Autodesk Inventor part; units mm, degrees
ref_plane "YZ Plane" through (0, 0, 0) normal (1, 0, 0) x (0, 1, 0)
ref_plane "XZ Plane" through (0, 0, 0) normal (0, 1, 0) x (-1, 0, 0)
ref_plane "XY Plane" through (0, 0, 0) normal (0, 0, 1) x (1, 0, 0)
sketch "Sketch1" plane through (0, 0, 0) normal (0, 0, 1) x (1, 0, 0)
  circle A0 centre (-18.3721, 25.1477) radius 2.1844
  circle A1 centre (57.8279, 25.1477) radius 2.1844
  circle A2 centre (32.4279, -12.9523) radius 2.1844
  circle A3 centre (-56.4721, -12.9523) radius 2.1844
  arc A4 (-60.9623, -8.4622) -> (-56.4721, -19.3023) centre (-56.4721, -12.9523) ccw
  arc A5 (-18.3721, 31.4977) -> (-22.8623, 29.6378) centre (-18.3721, 25.1477) ccw
  line L0 (68.9404, 23.5133) -> (68.9404, 25.1477)
  line L1 (62.5904, 31.4977) -> (57.8279, 31.4977)
  arc A6 (68.9404, 25.1477) -> (62.5904, 31.4977) centre (62.5904, 25.1477) ccw
  line L2 (-3.5614, -19.3023) -> (-56.4721, -19.3023)
  line L3 (-60.9623, -8.4622) -> (-22.8623, 29.6378)
  line L4 (-18.3721, 31.4977) -> (57.8279, 31.4977)
  arc A7 (35.7428, -27.2531) -> (68.9404, 23.5133) centre (13.525, 23.5133) ccw
  line L5 (29.3044, -27.6849) -> (3.4241, -20.2818)
  arc A8 (29.3044, -27.6849) -> (35.7428, -27.2531) centre (31.9239, -18.5272) ccw
  arc A9 (3.4241, -20.2818) -> (-3.5614, -19.3023) centre (-3.5614, -44.7023) ccw
  point P0 (0, 0)
  point P1 (32.4279, -28.5784)
  dimension "d0" = 4.3688
  dimension "d1" = 12.7
  dimension "d2" = 12.7
  dimension "d4" = 6.35
  dimension "d21" = 9.525
  dimension "d22" = 25.4
extrude "Extrusion1" add sketch "Sketch1" along normal blind 1.5875
sketch "Sketch2" plane through (0, 0, 1.5875) normal (0, 0, 1) x (1, 0, 0)
  circle A0 centre (57.15, 0) radius 2.0828
  point P0 (0, 0)
  dimension "d7" = 4.1656
extrude "Extrusion2" cut sketch "Sketch2" against normal blind 1.5875
sketch "Sketch3" plane through (57.8279, 25.1477, 1.5875) normal (0, 0, 1) x (1, 0, 0)
  circle A0 centre (-50.8, 25.4) radius 2.0828
  arc A1 (-45.3375, 28.6378) -> (-55.2901, 29.8901) centre (-50.8, 25.4) ccw
  line L0 (-80.6901, 4.4901) -> (-55.2901, 29.8901)
  arc A2 (-76.2, 6.35) -> (-80.6901, 4.4901) centre (-76.2, 0) ccw
  arc A3 (-45.3375, 28.6378) -> (-6.2178, 6.35) centre (-6.2178, 51.8254) ccw
  line L1 (4.7625, 6.35) -> (-76.2, 6.35)
  dimension "d17" = 4.1656
extrude "Extrusion4" add sketch "Sketch3" against normal blind 1.5875
properties part number "sled" material "Acetal Resin, White"
Input: part model. Units: mm. Frame: model coordinates. Coordinates: 2 decimals unless noted, no trailing zeros. Loops run counter-clockwise (first coordinate to the right, second up) from the corner with the lowest first, then second, coordinate; pieces in that order, holes last.
Q1. Section C-C, the plane y = 0. Return the cut outline in (x, z).
Results are:
outline: (-52.5, 0) - (55.07, 0) - (55.07, 1.59) - (-52.5, 1.59) - close; (59.23, 0) - (63.7, 0) - (63.7, 1.59) - (59.23, 1.59) - close
Q2. Line query: line 1 along X through (y, z) = (26.5, 1.3); line 2 along Y through (x, z) = (-17.5, 1.1); line 3 along X through (y, z) = (50.5, 0.6). Output: solid intervals per line, ascending.
Results are:
line 1: x = -26 to -20.09, -16.66 to 56.11, 59.54 to 68.79
line 2: y = -19.3 to 23.14, 27.15 to 35
line 3: x = -2 to 4.95, 9.11 to 14.63
Q3. Section A-A, the plane x = 57.15. Return the cut outline in (y, z).
Results are:
outline: (-10.66, 0) - (-2.08, 0) - (-2.08, 1.59) - (-10.66, 1.59) - close; (2.08, 0) - (23.07, 0) - (23.07, 1.59) - (2.08, 1.59) - close; (27.22, 0) - (31.5, 0) - (31.5, 1.59) - (27.22, 1.59) - close
Q4. Mould query, pull axis X, two halves, no side actions, for faces 1 (the cylindrical face through (28.813, 37.625, 0.805)), 2 (the cylindrical face through (-62.298, -15.479, 0.783)), 3 (the cylindrical face through (55.07, 0.09, 0.8)). Classes: +X half, -X half, draft (parallel to the pull), parting line (faces both ways), or undercut.
Results are:
face 1: +X half
face 2: -X half
face 3: undercut
Q5. Section B-B, the plane z = 1.3. Return the cut outline in (x, y).
Results are:
outline: (-60.96, -8.46) arc R6.35 ccw to (-56.47, -19.3) - (-3.56, -19.3) arc R25.4 cw to (3.42, -20.28) - (29.3, -27.68) arc R9.53 ccw to (35.74, -27.25) arc R55.42 ccw to (68.94, 23.51) - (68.94, 25.15) arc R6.35 ccw to (62.59, 31.5) - (51.61, 31.5) arc R45.48 cw to (12.49, 53.79) arc R6.35 ccw to (2.54, 55.04) - close; hole circle Ø4.37 at (-56.47, -12.95); hole circle Ø4.37 at (-18.37, 25.15); hole circle Ø4.17 at (7.03, 50.55); hole circle Ø4.37 at (32.43, -12.95); hole circle Ø4.17 at (57.15, 0); hole circle Ø4.37 at (57.83, 25.15)
Q6. Contact query for a flat-ended pin moving along its axis: pin 1 (0.5 mm diameter, centred on x = 54.5, z = 0.5, fed in from +Y). Output: stop coordinate, or through.
Results are:
pin 1: stops at y = 31.5
Q7. Section D-D, the plane x = -26.5. Return the cut outline in (y, z), and give its area (3 significant figures).
Results are:
outline: (-19.3, 0) - (26, 0) - (26, 1.59) - (-19.3, 1.59) - close
area: 71.9 mm2
